```python
from build123d import *

# Parameters (mm, degrees)
F0_W     = 177.8
F0_H     = 152.4
F1_DEPTH = 50.8
F2_R     = 20.627653
F3_DEPTH = 161.036


with BuildPart() as f1:
    # F0 (on Top) → F1 (new body)
    with BuildSketch(Plane.XY):
        with Locations((13.166458, 42.614249)):
            Rectangle(F0_W, F0_H)
    extrude(amount=F1_DEPTH)

    # F2 (on face) → F3 (cut)
    with BuildSketch(Plane.YZ.offset(102.066458)):
        with Locations((-8.185751, 29.801123)):
            Circle(F2_R)
        with Locations((42.614249, 29.801123)):
            Circle(F2_R)
        with Locations((93.414249, 29.801123)):
            Circle(F2_R)
    extrude(amount=-F3_DEPTH, mode=Mode.SUBTRACT)


solid = f1.part
```
Could you check a few things on this model? Use its own coordinates, in mm. A direction names the side the tool comes from. Give positions to 0.01 mm unless a question says otherwise; leave off trailing zeros. Loops run counter-clockwise (first coordinate to the right, second up) from the corner with the lowest first, then second, coordinate; pieces in that order, holes last. Notation, with made-up numbers: (81, -9) - (108, -9) arc R14 ccw to (108, 9) - close; hole circle Ø3 at (5.25, 36). An arc over 180 degrees is marked (long way). Answer in a Markdown table with one row per item. Add a question column.
Q1. If we section it at D-D (y = 7): List the corners of the cut face in (x, z) for me.
Q2. Which directions (+Z, -Z, +X, -X, +Y, -Y) give clear straight access to the entire face, cutting with the end or side of a thin tool? Please do faces 4 (the face through (12, -33.586, 25)), 5 (the face through (-58.97, 93, 30)).
Q3. Please list where these lines run through material, in increasing order: L1, parallel to Y at x = -58, z = 30.5; L2, parallel to Y at x = 30.5, z = 19.5; L3, parallel to X at y = 105.5, z = 29. Write a range as from..to.
Q4. If we section it at B-B (y = 47.5): List the corners of the cut face in (x, z) for me, plus the area to 3 significant figures.
Q5. We'd pull the mould along Z, two halves only. Please class faces 1 (the face through (22.676, 22.007, 30.708)), 2 (the face through (-75.734, 42, 25)), 3 (the face through (12, 44, 0)): +Z half, -Z half, draft (parallel to the pull), parting line (faces both ways), or undercut.
Q6. If we section it at A-A (x = -22): List the corners of the cut face in (y, z) for me, plus the area to 3 significant figures.
Q7. If we section it at C-C (z = 39.5): List the corners of the cut face in (x, y) for me.
Q8. For pin 1 (20.5 mm diameter, centred on y = 35, z = 33, fed in from +X), with a flat end and sliding along its axis, tell me the tip position at first contact or that it passes through.
The answers:
| question | item | result |
|---|---|---|
| 1 | outline | (-75.73, 0) - (102.07, 0) - (102.07, 15.84) - (-58.97, 15.84) - (-58.97, 43.76) - (102.07, 43.76) - (102.07, 50.8) - (-75.73, 50.8) - close |
| 2 | face 4 | +Z, -Z, +X, -X, -Y |
| 2 | face 5 | +X |
| 3 | L1 | y = -33.59..-28.8, 12.43..22, 63.23..72.8, 114.03..118.81 |
| 3 | L2 | y = -33.59..-26.06, 9.69..24.74, 60.49..75.54, 111.29..118.81 |
| 3 | L3 | x = -75.73..-58.97 |
| 4 | outline | (-75.73, 0) - (102.07, 0) - (102.07, 9.76) - (-58.97, 9.76) - (-58.97, 49.84) - (102.07, 49.84) - (102.07, 50.8) - (-75.73, 50.8) - close |
| 4 | area | 2,580 mm^2 |
| 5 | face 1 | undercut |
| 5 | face 2 | draft |
| 5 | face 3 | -Z half |
| 6 | outline | (-33.59, 0) - (118.81, 0) - (118.81, 50.8) - (-33.59, 50.8) - close; hole circle Ø41.26 at (-8.19, 29.8); hole circle Ø41.26 at (42.61, 29.8); hole circle Ø41.26 at (93.41, 29.8) |
| 6 | area | 3,730 mm^2 |
| 7 | outline | (-75.73, -33.59) - (102.07, -33.59) - (102.07, -26.39) - (-58.97, -26.39) - (-58.97, 10.02) - (102.07, 10.02) - (102.07, 24.41) - (-58.97, 24.41) - (-58.97, 60.82) - (102.07, 60.82) - (102.07, 75.21) - (-58.97, 75.21) - (-58.97, 111.62) - (102.07, 111.62) - (102.07, 118.81) - (-75.73, 118.81) - close |
| 8 | pin 1 | stops at x = -58.97 |
